Geometry: final body of the model. Coordinates: model frame, mm. A direction names the side the tool comes from. Give positions to 0.01 mm unless a question says otherwise; leave off trailing zeros. Loops run counter-clockwise (first coordinate to the right, second up) from the corner with the lowest first, then second, coordinate; pieces in that order, holes last.
1. Section C-C, the plane z = -5. Output: boundary loops of the cut face in (x, y).
2. Section A-A, the plane x = -7.5. Output: boundary loops of the cut face in (y, z), then the cut area to 3 significant figures.
3. Material intervals for line 1 along X through (y, z) = (21, -4.25); line 2 along X through (y, z) = (23, -3.75); line 3 along Y through (x, z) = (-18.5, -5), sorted ascending.
4. Section D-D, the plane y = 58.5. Output: boundary loops of the cut face in (x, z).
5. Section B-B, the plane y = 35. Output: boundary loops of the cut face in (x, z).
6. Draft query along X for faces 3 (the face through (20.584, 45, -5)), 4 (the face through (-69.416, 18, -5)), 5 (the face through (-18.19, 18.62, -4.93)). Return one class per face: +X half, -X half, draft (parallel to the pull), parting line (faces both ways), or undercut.
7. Access query for faces 1 (the face through (-19, 10.892, -5)), 2 (the face through (-51.916, 45, -5)). Directions: +Z, -Z, +X, -X, +Y, -Y. A direction counts if a zero-diameter tool reaches every point of the face in a straight line with its end or side. Return the directions, or none.
8. First-contact query: P1, Ø5, axis at x = 13.5, y = 41.5, coming from the +Z side; P2, Ø6, axis at y = 44.5, z = -1.5, coming from the +X side; P3, Ø3, axis at x = -63, z = -3, coming from the +Y side; P4, Ø3, axis at y = 55, z = -8, coming from the +X side. Flat tips, straight axial feed; report the tip coordinate or a pass-through.
Autodesk Inventor part; units mm, degrees
ref_plane "YZ Plane" through (0, 0, 0) normal (1, 0, 0) x (0, 1, 0)
ref_plane "XZ Plane" through (0, 0, 0) normal (0, 1, 0) x (-1, 0, 0)
ref_plane "XY Plane" through (0, 0, 0) normal (0, 0, 1) x (1, 0, 0)
sketch "Sketch1" plane through (0, 0, 0) normal (0, 0, 1) x (1, 0, 0)
  line L0 (30.5843, 30.8924) -> (30.5843, 10.8924)
  line L1 (30.5843, 10.8924) -> (-69.4157, 10.8924)
  line L2 (-69.4157, 10.8924) -> (-69.4157, 31.1924)
  line L3 (-69.4157, 21.0424) -> (30.5843, 20.8924) construction
  line L4 (-9.4157, 61.1924) -> (-39.4157, 61.1924)
  line L5 (-51.9157, 48.6924) -> (-51.9157, 41.1924)
  arc A0 (-39.4157, 61.1924) -> (-51.9157, 48.6924) centre (-39.4157, 48.6924) ccw
  line L6 (30.5843, 30.8924) -> (30.5843, 30.8924)
  line L7 (-61.9157, 31.1924) -> (-69.4157, 31.1924)
  arc A1 (-61.9157, 31.1924) -> (-51.9157, 41.1924) centre (-61.9157, 41.1924) ccw
  circle A2 centre (-19.4157, 20.9674) radius 2.65
  line L8 (-69.4157, 21.0424) -> (-19.4157, 20.9674) construction
  line L9 (-19.4157, 20.9674) -> (30.5843, 20.8924) construction
  circle A3 centre (-44.4157, 21.0049) radius 2.65
  circle A4 centre (5.5843, 20.9299) radius 2.65
  line L10 (-9.4157, 51.1924) -> (-9.4157, 30.8924) construction
  line L11 (-9.4157, 51.1924) -> (-9.4157, 30.8924) construction
  circle A5 centre (-9.4157, 41.0424) radius 10.15
  line L12 (-9.4157, 61.1924) -> (8.0843, 61.1924)
  line L13 (20.5843, 48.6924) -> (20.5843, 40.8924)
  arc A6 (20.5843, 48.6924) -> (8.0843, 61.1924) centre (8.0843, 48.6924) ccw
  arc A7 (20.5843, 40.8924) -> (30.5843, 30.8924) centre (30.5843, 40.8924) ccw
  point P0 (0, 0)
  point P1 (20.5843, 61.1924)
  point P2 (30.5843, 30.8924)
  dimension "d0" = 100
  dimension "d1" = 20
  dimension "d2" = 20.3
  dimension "d6" = 10
  dimension "d9" = 12.5
  dimension "d10" = 30
  dimension "d11" = 10
  dimension "d12" = 40
  dimension "d13" = 5.3
  dimension "d14" = 5.3
  dimension "d15" = 5.3
  dimension "d18" = 30
  dimension "d19" = 12.5
  dimension "d20" = 10
extrude "Extrusion1" add sketch "Sketch1" against normal blind 10
fillet "Fillet1" radius 5 2 edges at (-69.4157, 31.1924, -5) (30.5843, 30.8924, -5)
properties part number "bottomhingeholder"
Answers below:
1. outline: (-69.42, 10.89) - (30.58, 10.89) - (30.58, 26.75) arc R5 ccw to (27.25, 31.46) arc R10 cw to (20.58, 40.89) - (20.58, 48.69) arc R12.5 ccw to (8.08, 61.19) - (-39.42, 61.19) arc R12.5 ccw to (-51.92, 48.69) - (-51.92, 41.19) arc R10 cw to (-61.92, 31.19) - (-64.42, 31.19) arc R5 ccw to (-69.42, 26.19) - close; hole circle Ø5.3 at (-44.42, 21); hole circle Ø5.3 at (-19.42, 20.97); hole circle Ø20.3 at (-9.42, 41.04); hole circle Ø5.3 at (5.58, 20.93)
2. outline: (10.89, -10) - (31.07, -10) - (31.07, 0) - (10.89, 0) - close; (51.01, -10) - (61.19, -10) - (61.19, 0) - (51.01, 0) - close
2. area: 304 mm2
3. line 1: x = -69.42 to -47.07, -41.77 to -22.07, -16.77 to 2.94, 8.23 to 30.58
3. line 2: x = -69.42 to -46.16, -42.67 to -21.12, -17.72 to 3.93, 7.24 to 30.58
3. line 3: y = 10.89 to 18.48, 23.45 to 36.51, 45.57 to 61.19
4. outline: (-47.17, -10) - (15.83, -10) - (15.83, 0) - (-47.17, 0) - close
5. outline: (-54.06, -10) - (-17.57, -10) - (-17.57, 0) - (-54.06, 0) - close; (-1.26, -10) - (22.5, -10) - (22.5, 0) - (-1.26, 0) - close
6. face 3: +X half
6. face 4: -X half
6. face 5: undercut
7. face 1: +Z, -Z, +X, -X, -Y
7. face 2: +Z, -Z, -X, +Y
8. P1: stops at z = 0
8. P2: stops at x = 20.58
8. P3: stops at y = 31.2
8. P4: stops at x = 19.62
